Verification items for the finished model (mm, model axes). Face numbers are marked on the shaded views. A direction names the side the tool comes from. Round coordinates to 2 decimals unless told otherwise and drop trailing zeros. Write each loop counter-clockwise with the first axis right and the second up, starting at its lowest first coordinate (ties: lowest second). Pieces come first, ordered by that corner, then holes. Notation, with made-up numbers: M -35,58.5 L -13,58.5 A28 cw -13,85.5 Z; hole C 48.25,52.5 d11. An arc over 180 degrees is marked long. One line per item, written item: value. Start each with the question number.
Item 1: Section check C-C, the plane z = 5.75. Record the cut outline in (x, y).
Item 2: Tool access check on the marked faces 1 and 2. Record the directions out of +Z, -Z, +X, -X, +Y, -Y that give a thin tool (end or side, any length) a straight path to the whole face; none if there is none.
Item 3: Section check B-B, the plane z = 1.5. Record the cut outline in (x, y).
Item 4: Thickness scan on probe 1 along Y at (x, z) = (-25, 1.65); probe 2 along X at (y, z) = (-2.25, 4); probe 3 along Z at (x, y) = (-40.5, 4.25). Record the ranges inside material, lowest first. Write a range as from..to.
Item 5: Section check A-A, the plane x = 25. Record the cut outline in (y, z).
Item 6: Section check D-D, the plane x = -27.5. Record the cut outline in (y, z), then the cut area to 4 significant figures.
Item 7: Gauge pin test, flat ends, axial feed: pin 1 (4 mm diameter, centred on y = 5.5, z = 3.5, fed in from +X); pin 2 (3 mm diameter, centred on x = 25, y = 0, fed in from +Z); pin 3 (0.6 mm diameter, centred on x = -16, y = -1, fed in from +Z). Record the tip position at first contact, or that the pin passes through.
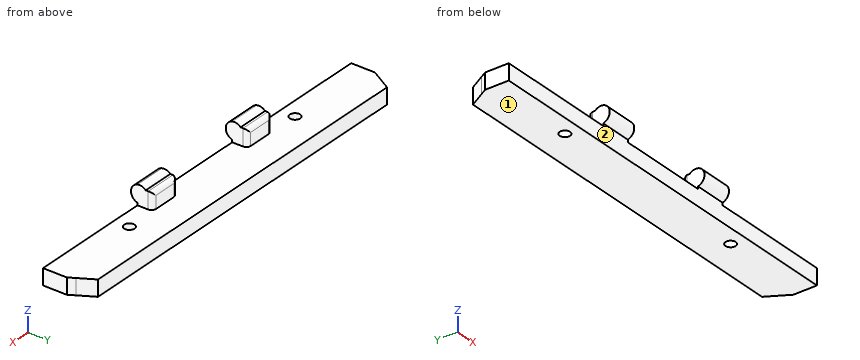
from build123d import *

# Parameters (mm, degrees)
SKETCH_1_W          = 93
SKETCH_1_H          = 7
SKETCH_1_R          = 1.2
EXTRUDE_1_DEPTH     = 3.7
SKETCH_2_W          = 7.4
SKETCH_2_H          = 3.5
EXTRUDE_2_DEPTH     = 5
EXTRUDE_3_DEPTH     = 7.4
EXTRUDE_START       = -7.4
EXTRUDE_4_DEPTH     = 7.4
CUT_EXTRUDE_1_DEPTH = 48.03456176
EXTRUDE_5_DEPTH     = 3.7
CUT_EXTRUDE_2_DEPTH = 66.459453099
FILLET_1_R          = 1


with BuildPart() as part:
    # ｽｹｯﾁ1 → ﾎﾞｽ - 押し出し1 (new body)
    with BuildSketch(Plane.XY):
        Rectangle(SKETCH_1_W, SKETCH_1_H)
        with Locations((-25, 0)):
            Circle(SKETCH_1_R, mode=Mode.SUBTRACT)
        with Locations((25, 0)):
            Circle(SKETCH_1_R, mode=Mode.SUBTRACT)
    extrude(amount=EXTRUDE_1_DEPTH)

    # ｽｹｯﾁ2 → ﾎﾞｽ - 押し出し2 (add)
    with BuildSketch(Plane.XY.offset(3.7)):
        with Locations((-14.3, -1.75)):
            Rectangle(SKETCH_2_W, SKETCH_2_H)
        with Locations((14.3, -1.75)):
            Rectangle(SKETCH_2_W, SKETCH_2_H)
    extrude(amount=EXTRUDE_2_DEPTH)

    # ｽｹｯﾁ3 → ﾎﾞｽ - 押し出し3 (add)
    with BuildSketch(Plane.ZY.offset(18)):
        with BuildLine():
            Line((4.263508327, -3.5), (8.136491673, -3.5))
            ThreePointArc((8.136491673, -3.5), (6.2, -5), (4.263508327, -3.5))
        make_face()
    extrude(amount=-EXTRUDE_3_DEPTH)

    # ｽｹｯﾁ4 → ﾎﾞｽ - 押し出し4 (add)
    with BuildSketch(Plane(origin=(18, 0, 0), x_dir=(0, 0, -1), z_dir=(1, 0, 0)).offset(EXTRUDE_START)):
        with BuildLine():
            Line((-8.136491673, -3.5), (-4.263508327, -3.5))
            ThreePointArc((-4.263508327, -3.5), (-6.2, -5), (-8.136491673, -3.5))
        make_face()
    extrude(amount=EXTRUDE_4_DEPTH)

    # ｽｹｯﾁ5 → ｶｯﾄ - 押し出し1 (cut, through all)
    with BuildSketch(Plane.XY.offset(3.7)):
        Polygon((-46.5, 2), (-45.633974596, 3.5), (-46.5, 3.5), align=None)
        Polygon((46.5, 3.5), (46.5, 2), (45.633974596, 3.5), align=None)
    extrude(amount=-CUT_EXTRUDE_1_DEPTH, mode=Mode.SUBTRACT)

    # ｽｹｯﾁ6 → ﾎﾞｽ - 押し出し5 (add)
    with BuildSketch(Plane.XY.offset(3.7)):
        Polygon((-45.633974596, 3.5), (45.633974596, 3.5), (43.613248654, 7), (-43.613248654, 7), align=None)
    extrude(amount=-EXTRUDE_5_DEPTH)

    # ｽｹｯﾁ7 → ｶｯﾄ - 押し出し2 (cut, through all)
    with BuildSketch(Plane(origin=(18, 0, 0), x_dir=(0, 0, -1), z_dir=(1, 0, 0))):
        with BuildLine():
            Line((-7.601258538, -1.572949017), (-7.601258538, 0))
            Line((-7.601258538, 0), (-8.7, 0))
            Line((-8.7, 0), (-8.7, -3.5))
            Line((-8.7, -3.5), (-8.136491673, -3.5))
            ThreePointArc((-8.136491673, -3.5), (-8.127050983, -2.464766865), (-7.601258538, -1.572949017))
        make_face()
    extrude(amount=-CUT_EXTRUDE_2_DEPTH, mode=Mode.SUBTRACT)

    # ﾌｨﾚｯﾄ1
    fillet_1_edges = [part.edges().sort_by_distance(p)[0] for p in [
        (10.6, 0, 5.650629269),
        (18, 0, 5.650629269),
        (-18, 0, 5.650629269),
        (-10.6, 0, 5.650629269),
        (-14.3, 0, 7.601258538),
        (14.3, 0, 7.601258538),
    ]]
    fillet(fillet_1_edges, radius=FILLET_1_R)


solid = part.part
Response values:
1. outline: M -18,-4.95 L -10.6,-4.95 L -10.6,-1 A1 ccw -11.6,0 L -17,0 A1 ccw -18,-1 Z; M 10.6,-4.95 L 18,-4.95 L 18,-1 A1 ccw 17,0 L 11.6,0 A1 ccw 10.6,-1 Z
2. face 1: -Z, +X, -X, +Y, -Y
2. face 2: -Z, +X, -X, -Y
3. outline: M -46.5,-3.5 L 46.5,-3.5 L 46.5,2 L 43.61,7 L -43.61,7 L -46.5,2 Z; hole C -25,0 d2.4; hole C 25,0 d2.4
4. probe 1: y = -3.5..-1.2, 1.2..7
4. probe 2: x = -18..-10.6, 10.6..18
4. probe 3: z = 0..3.7
5. outline: M -3.5,0 L -1.2,0 L -1.2,3.7 L -3.5,3.7 Z; M 1.2,0 L 7,0 L 7,3.7 L 1.2,3.7 Z
6. outline: M -3.5,0 L 7,0 L 7,3.7 L -3.5,3.7 Z
6. area: 38.85 mm2
7. pin 1: stops at x = 45.63
7. pin 2: stops at z = 3.7
7. pin 3: stops at z = 7.6
